Verification items for the finished model (mm, model axes). Face numbers are marked on the shaded views. A direction names the side the tool comes from. Round coordinates to 2 decimals unless told otherwise and drop trailing zeros. Loops run counter-clockwise (first coordinate to the right, second up) from the corner with the lowest first, then second, coordinate; pieces in that order, holes last. Notation, with made-up numbers: M -15.5,54 L -3.5,54 A26 cw -3.5,69 Z; hole C 7,11 d1. An arc over 180 degrees is marked long. One line per item, written item: value.
from build123d import *

# Parameters (mm, degrees)
SKETCH1_W           = 75
SKETCH1_H           = 22.5
BOSS_EXTRUDE1_DEPTH = 18.5
SKETCH2_R           = 2.5
BOSS_EXTRUDE2_DEPTH = 10
SKETCH3_R           = 1.5
CUT_EXTRUDE1_DEPTH  = 15


with BuildPart() as part:
    # Sketch1 → Boss-Extrude1 (new body)
    with BuildSketch(Plane.XY):
        with Locations((40, -1.859504132)):
            Rectangle(SKETCH1_W, SKETCH1_H)
    extrude(amount=BOSS_EXTRUDE1_DEPTH)

    # Sketch2 → Boss-Extrude2 (add)
    with BuildSketch(Plane.XY.offset(18.5)):
        with Locations(Location((66.5, -2.437272613, 0), (0, 0, 180))):
            Circle(SKETCH2_R)
    extrude(amount=BOSS_EXTRUDE2_DEPTH)

    # Sketch3 → Cut-Extrude1 (cut)
    with BuildSketch(Plane(origin=(0, 0, 0), x_dir=(-1, 0, 0), z_dir=(0, 0, -1))):
        with Locations((-46, 7.390495868)):
            Circle(SKETCH3_R)
        with Locations((-46, -11.109504132)):
            Circle(SKETCH3_R)
    extrude(amount=-CUT_EXTRUDE1_DEPTH, mode=Mode.SUBTRACT)


solid = part.part
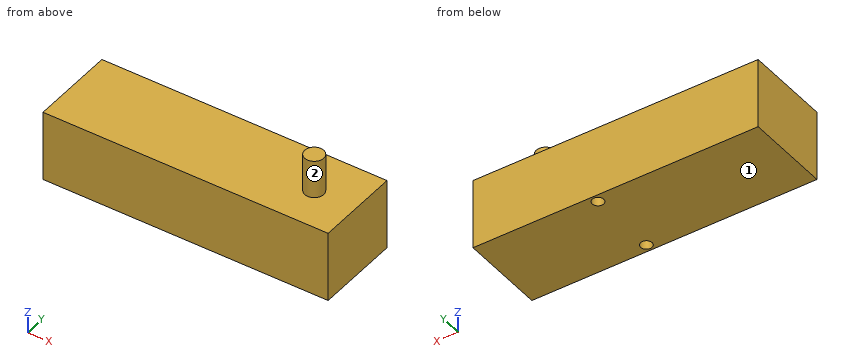
(1) Sectioned sample at C-C on x = 58.5. Enter the section's corners in (y, z).
Completed:
outline: M -13.11,0 L 9.39,0 L 9.39,18.5 L -13.11,18.5 Z
(2) Tool access check on the marked faces 1 and 2. Record the directions out of +Z, -Z, +X, -X, +Y, -Y that give a thin tool (end or side, any length) a straight path to the whole face; none if there is none.
Completed:
face 1: -Z, +X, -X, +Y, -Y
face 2: +Z
(3) Depth check by flat-ended pin: pin 1 Ø1.8 at (x, y) = (46, 7.39) entering from -Z; pin 2 Ø12 at (y, z) = (3, 25.5) entering from -X; pin 3 Ø3 at (y, z) = (-6.5, 20.5) entering from +X. Enter the tip coordinate at first touch or a pass-through.
Completed:
pin 1: stops at z = 15
pin 2: stops at x = 64
pin 3: passes through
(4) Thickness scan on L1, parallel to Y at x = 46, z = 6; L2, parallel to Y at x = 45, z = 10.5; L3, parallel to Z at x = 13.5, y = -1. Record the ranges inside material, lowest first. Write a range as from..to.
Completed:
L1: y = -13.11..-12.61, -9.61..5.89, 8.89..9.39
L2: y = -13.11..-12.23, -9.99..6.27, 8.51..9.39
L3: z = 0..18.5
(5) Sectioned sample at B-B on y = -7.75. Enter the section's corners in (x, z).
Completed:
outline: M 2.5,0 L 77.5,0 L 77.5,18.5 L 2.5,18.5 Z
(6) Sectioned sample at A-A on x = 66.5. Enter the section's corners in (y, z), and give its area (3 significant figures).
Completed:
outline: M -13.11,0 L 9.39,0 L 9.39,18.5 L 0.06,18.5 L 0.06,28.5 L -4.94,28.5 L -4.94,18.5 L -13.11,18.5 Z
area: 466 mm^2
